from build123d import *

# Parameters (mm, degrees)
EXTRUDE_1_DEPTH = 12
SKETCH_2_W      = 18
SKETCH_2_H      = 18
EXTRUDE_2_DEPTH = 6
EXTRUDE_3_DEPTH = 10


with BuildPart() as part:
    # 스케치1 → 보스-돌출1 (new body)
    with BuildSketch(Plane.XY):
        with BuildLine():
            Line((15.355510937, 5.870718563), (-16.644489063, 5.870718563))
            Line((-16.644489063, 5.870718563), (-16.644489063, -6.129281437))
            Line((-16.644489063, -6.129281437), (-9.139386491, -6.129281437))
            ThreePointArc((-9.139386491, -6.129281437), (1.71732924, 2.709540377), (15.355510937, 5.870718563))
        make_face()
    extrude(amount=EXTRUDE_1_DEPTH)

    # 스케치2 → 보스-돌출2 (add)
    with BuildSketch(Plane.ZY.offset(16.644489063)):
        with Locations((6, -0.129281437)):
            Rectangle(SKETCH_2_W, SKETCH_2_H)
    extrude(amount=EXTRUDE_2_DEPTH)

    # 스케치3 → 보스-돌출3 (add)
    with BuildSketch(Plane.ZY.offset(22.644489063)):
        with BuildLine():
            Line((5.428283523, 1.573651364), (5.428283523, 2.573651364))
            Line((5.428283523, 2.573651364), (7.272757062, 2.573651364))
            Line((7.272757062, 2.573651364), (7.272757062, 1.573651364))
            ThreePointArc((7.272757062, 1.573651364), (6.645038385, -0.426348636), (7.272757062, -2.426348636))
            Line((7.272757062, -2.426348636), (5.428283523, -2.426348636))
            ThreePointArc((5.428283523, -2.426348636), (6.0560022, -0.426348636), (5.428283523, 1.573651364))
        make_face()
    extrude(amount=EXTRUDE_3_DEPTH)


solid = part.part
Model file for the job. Use its own axes, mm. A direction names the side the tool comes from. Give positions to 0.01 mm unless a question says otherwise; leave off trailing zeros. Loops run counter-clockwise (first coordinate to the right, second up) from the corner with the lowest first, then second, coordinate; pieces in that order, holes last. Notation, with made-up numbers: (78, 50.5) -> (124, 50.5) arc R19 cw to (124, 85.5) -> close; hole circle Ø6 at (77.25, -31). An arc over 180 degrees is marked (long way). Use a Markdown table: item, result. Add a question column.
(1) Slice it at C-C on x = -27.5. List the corners of the cut face in (y, z), and give its area (3 significant figures).
(2) Slice it at A-A on z = 3.75. List the corners of the cut face in (x, y).
(3) Slice it at B-B on y = -1. List the corners of the cut face in (x, z).
(4) Wall check: line 1 along Z through (x, y) = (-28, 2.25); line 2 along X through (y, z) = (7.25, -1.5); line 3 along Y through (x, z) = (-13, 11.25). Give the ranges that are in metal, low to high.
(5) Mould opens along Y. For faces 6 (the cylindrical face through (-27.574, -0.397, 6.645)), 7 (the flat face through (-20, 0, -3)), 8 (the flat face through (-28, -2.426, 6)) say: +Y half, -Y half, draft (parallel to the pull), parting line (faces both ways), or undercut.
(6) Slice it at D-D on y = 3.5. List the corners of the cut face in (x, z).
(7) Tool access for faces 1 (the flat face through (0, 5.871, 6)), 2 (the flat face through (-13, -6.129, 6)), 3 (the flat face through (-28, 2, 7.273)), 4 (the flat face through (-28, 2.574, 6)), 5 (the flat face through (-28, 2, 5.428)): list every direction of +Z, -Z, +X, -X, +Y, -Y with a clear straight run to the whole face (end or side of a thin tool).
(8) Drop flat-ended pins along their axis: pin 1 Ø1.1 at (x, y) = (-28, 2) entering from -Z; pin 2 Ø5 at (x, z) = (-8, 6.5) entering from -Y; pin 3 Ø6 at (x, y) = (-6.5, 1) entering from +Z. Give the stop position or say it passes through.
Filled sheet:
| question | item | result |
|---|---|---|
| 1 | outline | (-2.43, 5.43) arc R3.5 cw to (1.57, 5.43) -> (2.57, 5.43) -> (2.57, 7.27) -> (1.57, 7.27) arc R3.5 cw to (-2.43, 7.27) -> close |
| 1 | area | 5.81 mm2 |
| 2 | outline | (-22.64, -9.13) -> (-16.64, -9.13) -> (-16.64, -6.13) -> (-9.14, -6.13) arc R31 cw to (15.36, 5.87) -> (-16.64, 5.87) -> (-16.64, 8.87) -> (-22.64, 8.87) -> close |
| 3 | outline | (-32.64, 6.01) -> (-22.64, 6.01) -> (-22.64, -3) -> (-16.64, -3) -> (-16.64, 0) -> (-4.11, 0) -> (-4.11, 12) -> (-16.64, 12) -> (-16.64, 15) -> (-22.64, 15) -> (-22.64, 6.69) -> (-32.64, 6.69) -> close |
| 4 | line 1 | 5.43 to 7.27 |
| 4 | line 2 | -22.64 to -16.64 |
| 4 | line 3 | -6.13 to 5.87 |
| 5 | face 6 | undercut |
| 5 | face 7 | draft |
| 5 | face 8 | -Y half |
| 6 | outline | (-22.64, -3) -> (-16.64, -3) -> (-16.64, 0) -> (3.47, 0) -> (3.47, 12) -> (-16.64, 12) -> (-16.64, 15) -> (-22.64, 15) -> close |
| 7 | face 1 | +Z, -Z, +X, +Y |
| 7 | face 2 | +Z, -Z, +X, -Y |
| 7 | face 3 | +Z, -X, +Y, -Y |
| 7 | face 4 | +Z, -Z, -X, +Y |
| 7 | face 5 | -Z, -X, +Y, -Y |
| 8 | pin 1 | z = 5.43 |
| 8 | pin 2 | y = -6.13 |
| 8 | pin 3 | z = 12 |
